Geometry check sheet. Reference: drawing and pictorial views, mm from the part's lowest x, y, z. A direction names the side the tool comes from. Round coordinates to 2 decimals unless told otherwise and drop trailing zeros. Order: outer loops, then holes, each group sorted by start corner. A loop starts at its lowest first (then second) coordinate and runs counter-clockwise, first axis right, second up. Notation, with made-up numbers: (-22.75, -19) -> (15.25, -19) arc R21 ccw to (15.25, 8) -> close; hole circle Ø11 at (-28, -23.75). An arc over 180 degrees is marked (long way). Put each result on its own line as item: value.
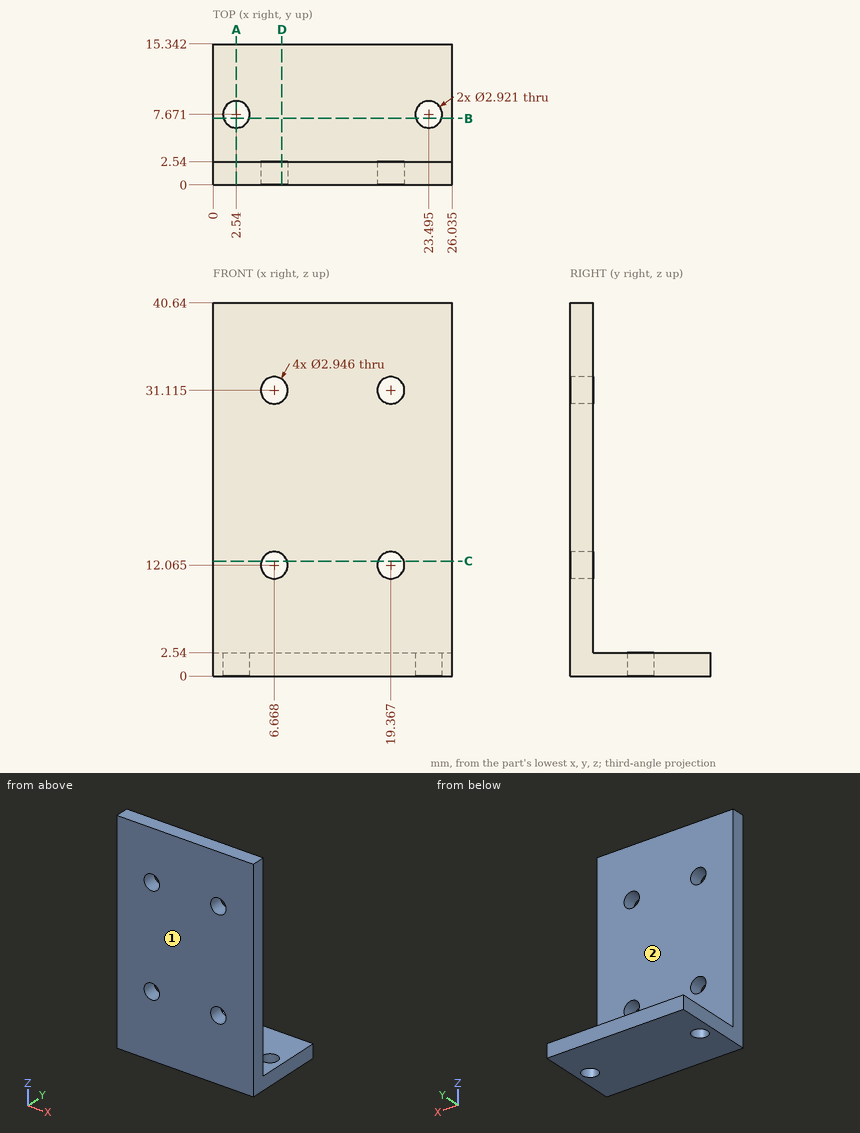
Item 1: Sectioned sample at A-A, the plane x = 2.54. Record the boundary of the cut face in (y, z).
Geometry check:
outline: (0, 0) -> (6.21, 0) -> (6.21, 2.54) -> (2.54, 2.54) -> (2.54, 40.64) -> (0, 40.64) -> close; (9.13, 0) -> (15.34, 0) -> (15.34, 2.54) -> (9.13, 2.54) -> close
Item 2: Sectioned sample at D-D, the plane x = 7.5. Record the boundary of the cut face in (y, z).
Geometry check:
outline: (0, 0) -> (15.34, 0) -> (15.34, 2.54) -> (2.54, 2.54) -> (2.54, 10.85) -> (0, 10.85) -> close; (0, 13.28) -> (2.54, 13.28) -> (2.54, 29.9) -> (0, 29.9) -> close; (0, 32.33) -> (2.54, 32.33) -> (2.54, 40.64) -> (0, 40.64) -> close
Item 3: Depth check by flat-ended pin: pin 1 Ø3.5 at (x, y) = (2.54, 7.67) entering from +Z; pin 2 Ø13 at (x, z) = (11.5, 23) entering from +Y. Enter the tip coordinate at first touch or a pass-through.
Geometry check:
pin 1: z = 2.54
pin 2: y = 2.54
Item 4: Material ranges on line 1 along Z through (x, y) = (21.75, 8.75), recorded low to high.
Geometry check:
line 1: 0 to 2.54
Item 5: Tool access check on the marked faces 1 and 2. Record the directions out of +Z, -Z, +X, -X, +Y, -Y that give a thin tool (end or side, any length) a straight path to the whole face; none if there is none.
Geometry check:
face 1: +Z, -Z, +X, -X, -Y
face 2: +Z, +X, -X, +Y
Item 6: Sectioned sample at C-C, the plane z = 12.5. Record the boundary of the cut face in (x, y) (1 decimal).
Geometry check:
outline: (0, 0) -> (5.3, 0) -> (5.3, 2.5) -> (0, 2.5) -> close; (8.1, 0) -> (18, 0) -> (18, 2.5) -> (8.1, 2.5) -> close; (20.8, 0) -> (26, 0) -> (26, 2.5) -> (20.8, 2.5) -> close
Item 7: Sectioned sample at B-B, the plane y = 7.25. Record the boundary of the cut face in (x, z) (1 decimal).
Geometry check:
outline: (0, 0) -> (1.1, 0) -> (1.1, 2.5) -> (0, 2.5) -> close; (3.9, 0) -> (22.1, 0) -> (22.1, 2.5) -> (3.9, 2.5) -> close; (24.9, 0) -> (26, 0) -> (26, 2.5) -> (24.9, 2.5) -> close
